Check sheet for the modelled part. Datum: model origin and axes. Units: mm. A direction names the side the tool comes from. Coordinates: 2 decimals unless noted, no trailing zeros. Loops run counter-clockwise (first coordinate to the right, second up) from the corner with the lowest first, then second, coordinate; pieces in that order, holes last. Notation, with made-up numbers: M 9.5,-13 L 47.5,-13 A26 ccw 47.5,12 Z; hole C -10,14.25 d5. An arc over 180 degrees is marked long. Use CSV: the item, a comma, the result in double quotes. Start each with the question number.
(1) Go/stop test with flat-tipped pins: pin 1 Ø3 at (x, z) = (2, 6.5) entering from -Y; pin 2 Ø0.6 at (x, y) = (1.5, 6) entering from -Z; pin 3 Ø0.6 at (y, z) = (-2, 0) entering from -X. Record where each tip stops, or that it passes through.
(2) Section check C-C on y = 3. Record the cut outline in (x, z) (3 decimals).
(3) Set-up check for faces 1 (the flat face through (0, 1, -3.3)), 2 (the flat face through (0, 5.7, 6)): record each of +Z, -Z, +X, -X, +Y, -Y from which the full face is reachable in a straight line by a thin tool's end or side.
(4) Section check D-D on z = 5.5. Record the cut outline in (x, y), and give its area (3 significant figures).
(5) Section check B-B on x = 0. Record the cut outline in (y, z) (3 decimals), and give its area (3 significant figures).
(6) Section check A-A on y = -0.75. Record the cut outline in (x, z).
(7) Scan lines: line 1 (Z direction, x = -1.45, y = -1.25); line 2 (Y direction, x = -0.2, z = 3.25); line 3 (Z direction, x = 2.75, y = 0.75). Record each from-to range of solid material in increasing order.
from build123d import *

# Parameters (mm, degrees)
BOSS_EXTRUDE1_DEPTH = 3
SKETCH3_W           = 0.5
SKETCH3_H           = 0.5
BOSS_EXTRUDE2_DEPTH = 3.175


with BuildPart() as part:
    # Sketch1 → Boss-Extrude1 (new body, symmetric)
    with BuildSketch(Plane(origin=(0, 0, 0), x_dir=(0, 0, -1), z_dir=(1, 0, 0))):
        Polygon((-6, 6), (-6, 0), (3.3, 0), (3.3, 1.5), (-0.25, 5.5), (-0.25, 6), align=None)
    extrude(amount=BOSS_EXTRUDE1_DEPTH, both=True)

    # Sketch2 → Revolve1 (revolve)
    with BuildSketch(Plane(origin=(0, 0, 0), x_dir=(0, 0, -1), z_dir=(1, 0, 0))):
        with BuildLine():
            Line((-6, 3), (-10.7, 3))
            ThreePointArc((-10.7, 3), (-9.989733944, 4.714733944), (-8.275, 5.425))
            Line((-8.275, 5.425), (-6, 5.425))
            Line((-6, 5.425), (-6, 3))
        make_face()
    revolve(axis=Axis((0, 3, 6), (0, 0, 1)))

    # Sketch3 → Boss-Extrude2 (add)
    with BuildSketch(Plane.XZ):
        with Locations((-1.27, 0)):
            Rectangle(SKETCH3_W, SKETCH3_H)
        with Locations((1.27, 0)):
            Rectangle(SKETCH3_W, SKETCH3_H)
    extrude(amount=BOSS_EXTRUDE2_DEPTH)


solid = part.part
Outcome:
1,pin 1,"stops at y = 0"
1,pin 2,"stops at z = 0.25"
1,pin 3,"stops at x = -1.52"
2,outline,"M -3,-1.969 L 3,-1.969 L 3,6 L 2.425,6 L 2.425,8.275 A2.425 ccw -2.425,8.275 L -2.425,6 L -3,6 Z"
3,face 1,"-Z, +X, -X, +Y, -Y"
3,face 2,"+Z"
4,outline,"M -3,0 L 3,0 L 3,6 L -3,6 Z"
4,area,"36.0 mm²"
5,outline,"M 0,-3.3 L 1.5,-3.3 L 5.5,0.25 L 6,0.25 L 6,6 L 5.425,6 L 5.425,8.275 A2.425 ccw 0.575,8.275 L 0.575,6 L 0,6 Z"
5,area,"67.2 mm²"
6,outline,"M -1.52,-0.25 L -1.02,-0.25 L -1.02,0.25 L -1.52,0.25 Z; M 1.02,-0.25 L 1.52,-0.25 L 1.52,0.25 L 1.02,0.25 Z"
7,line 1,"z = -0.25 to 0.25"
7,line 2,"y = 0 to 6"
7,line 3,"z = -3.3 to 6"
